from build123d import *

# Parameters (mm, degrees)
BOSS_EXTRUDE1_DEPTH     = 2.5
SKETCH2_W               = 2.5
SKETCH2_H               = 47.5
BOSS_EXTRUDE2_DEPTH     = 20
SKETCH3_W               = 2.5
SKETCH3_H               = 47.5
BOSS_EXTRUDE3_DEPTH     = 20
SKETCH4_W               = 17
SKETCH4_H               = 2.5
BOSS_EXTRUDE4_DEPTH     = 20.4
SKETCH5_W               = 1.5
SKETCH5_H               = 11
CUT_EXTRUDE1_DEPTH      = 48.5
SKETCH6_W               = 17
SKETCH6_H               = 2.5
BOSS_EXTRUDE5_DEPTH     = 20.4
SKETCH7_W               = 1.5
SKETCH7_H               = 11
CUT_EXTRUDE2_DEPTH      = 48.5
SKETCH8_W               = 2.7
SKETCH8_H               = 4.5
SKETCH9_W               = 2.7
SKETCH9_H               = 4.5
SKETCH10_W              = 2
SKETCH10_H              = 1.5
SKETCH11_W              = 2
SKETCH11_H              = 1.5
FILLET1_R               = 2
FILLET2_R               = 10
SKETCH13_R              = 3.6
SKETCH13_R_2            = 2.5
SKETCH13_R_3            = 1.5
CUT_EXTRUDE3_DEPTH      = 5.5
CUT_EXTRUDE3_DEPTH_BACK = 23.9


with BuildPart() as part:
    # Sketch1 → Boss-Extrude1 (new body)
    with BuildSketch(Plane(origin=(0, 0, 0), x_dir=(-1, 0, 0), z_dir=(0, 0, -1))):
        with BuildLine():
            Line((12, -20), (12, 32))
            Line((12, 32), (-12, 32))
            Line((-12, 32), (-12, -20))
            ThreePointArc((-12, -20), (0, -32), (12, -20))
        make_face()
    extrude(amount=-BOSS_EXTRUDE1_DEPTH)

    # Sketch2 → Boss-Extrude2 (add)
    with BuildSketch(Plane.ZY.offset(12)):
        with Locations((1.25, 8.25)):
            Rectangle(SKETCH2_W, SKETCH2_H)
    extrude(amount=BOSS_EXTRUDE2_DEPTH)

    # Sketch3 → Boss-Extrude3 (add)
    with BuildSketch(Plane(origin=(12, 0, 0), x_dir=(0, 0, -1), z_dir=(1, 0, 0))):
        with Locations((-1.25, 8.25)):
            Rectangle(SKETCH3_W, SKETCH3_H)
    extrude(amount=BOSS_EXTRUDE3_DEPTH)

    # Sketch4 → Boss-Extrude4 (add)
    with BuildSketch(Plane(origin=(0, 0, 0), x_dir=(-1, 0, 0), z_dir=(0, 0, -1))):
        with Locations((-23.5, -14.25)):
            Rectangle(SKETCH4_W, SKETCH4_H)
    extrude(amount=BOSS_EXTRUDE4_DEPTH)

    # Sketch5 → Cut-Extrude1 (cut, through all)
    with BuildSketch(Plane.XZ.offset(15.5)):
        with Locations((20.75, -14.9)):
            Rectangle(SKETCH5_W, SKETCH5_H)
    extrude(amount=-CUT_EXTRUDE1_DEPTH, mode=Mode.SUBTRACT)

    # Sketch6 → Boss-Extrude5 (add)
    with BuildSketch(Plane(origin=(0, 0, 0), x_dir=(-1, 0, 0), z_dir=(0, 0, -1))):
        with Locations((23.5, -14.25)):
            Rectangle(SKETCH6_W, SKETCH6_H)
    extrude(amount=BOSS_EXTRUDE5_DEPTH)

    # Sketch7 → Cut-Extrude2 (cut, through all)
    with BuildSketch(Plane.XZ.offset(15.5)):
        with Locations((-20.75, -14.9)):
            Rectangle(SKETCH7_W, SKETCH7_H)
    extrude(amount=-CUT_EXTRUDE2_DEPTH, mode=Mode.SUBTRACT)

    # Sketch8 → Revolve1 (revolve)
    with BuildSketch(Plane(origin=(0, 7.55, 0), x_dir=(1, 0, 0), z_dir=(0, 1, 0))):
        with Locations((10.85, -4.75)):
            Rectangle(SKETCH8_W, SKETCH8_H)
    revolve(axis=Axis((9.5, 7.55, 2.5), (0, 0, 1)))

    # Sketch9 → Revolve2 (revolve)
    with BuildSketch(Plane(origin=(0, 7.55, 0), x_dir=(1, 0, 0), z_dir=(0, 1, 0))):
        with Locations((24.85, -4.75)):
            Rectangle(SKETCH9_W, SKETCH9_H)
    revolve(axis=Axis((23.5, 7.55, 2.5), (0, 0, 1)))

    # Sketch10 → Revolve3 (revolve)
    with BuildSketch(Plane.XZ.offset(1.25)):
        with Locations((-18, -0.75)):
            Rectangle(SKETCH10_W, SKETCH10_H)
    revolve(axis=Axis((-19, -1.25, 0), (0, 0, -1)))

    # Sketch11 → Revolve4 (revolve)
    with BuildSketch(Plane.XZ.offset(-17.65)):
        with Locations((-0.5, -0.75)):
            Rectangle(SKETCH11_W, SKETCH11_H)
    revolve(axis=Axis((-1.5, 17.65, 0), (0, 0, -1)))

    # Fillet1
    fillet1_edges = [part.edges().sort_by_distance(p)[0] for p in [
        (32, -14.25, -20.4),
        (15, -14.25, -20.4),
        (-15, -14.25, -20.4),
        (-32, -14.25, -20.4),
    ]]
    fillet(fillet1_edges, radius=FILLET1_R)

    # Fillet2
    fillet2_edges = [part.edges().sort_by_distance(p)[0] for p in [
        (-32, 32, 1.25),
        (32, 32, 1.25),
    ]]
    fillet(fillet2_edges, radius=FILLET2_R)

    # Sketch13 → Cut-Extrude3 (cut, two sides)
    with BuildSketch(Plane.XY.offset(2.5)) as cut_extrude3_sk:
        with Locations((0, -20.1)):
            Circle(SKETCH13_R)
        with Locations((-20, 20.1)):
            Circle(SKETCH13_R_2)
        with Locations((-1.5, 17.65)):
            Circle(SKETCH13_R_3)
        with Locations((-19, -1.25)):
            Circle(SKETCH13_R_3)
        with Locations((9.5, 7.55)):
            Circle(SKETCH13_R_3)
        with Locations((23.5, 7.55)):
            Circle(SKETCH13_R_3)
    extrude(amount=CUT_EXTRUDE3_DEPTH, mode=Mode.SUBTRACT)
    extrude(cut_extrude3_sk.sketch, amount=-CUT_EXTRUDE3_DEPTH_BACK, mode=Mode.SUBTRACT)


solid = part.part
Design review of the part built by this model. Coordinates are the model's own, in mm. A direction names the side the tool comes from. Round coordinates to 2 decimals unless told otherwise and drop trailing zeros. Write each loop counter-clockwise with the first axis right and the second up, starting at its lowest first coordinate (ties: lowest second). Pieces come first, ordered by that corner, then holes. Notation, with made-up numbers: (9, 15.5) - (16, 15.5) arc R7 cw to (16, 23.5) - close; hole circle Ø11 at (21, 61). An arc over 180 degrees is marked (long way). Use a Markdown table: item, result. Add a question column.
1. Wall thickness on probe 1 along Y at (x, z) = (-20, 1.15); probe 2 along Y at (x, z) = (23.5, 5); probe 3 along X at (y, z) = (-14.5, -10): over which ranges is each line inside the solid? List them lowest first.
2. For faces 4 (the face through (21, -14, -9.4)), 5 (the face through (22, 6, 7)), 6 (the face through (-12, -18, 1)), 7 (the face through (12, -18, 1)), list the 3-axis set-ups (+Z, -Z, +X, -X, +Y, -Y) from which the entire face can be reached by the end or side of a thin tool; tool diameter is ignored.
3. We need section D-D (x = 23.5). State the section outline as (y, z) points.
4. We need section A-A (z = -14). State the section outline as (x, y) points, then the cut area to 3 significant figures.
5. We need section C-C (z = -4.5). State the section outline as (x, y) points.
6. Clearance check with flat-ended pins moving along their axes: pin 1 (2 mm diameter, centred on y = -18.5, z = 1, fed in from +X); pin 2 (19 mm diameter, centred on x = 4.5, y = -13.5, fed in from -Z); pin 3 (16 mm diameter, centred on x = -21.5, z = -11, fed in from -Y). State where each tip first meets the part, or that it passes through.
7. Mouldability with a two-part tool opening along Y and no side actions: class faces 1 (the face through (-0.47, -16.53, 1.27)), 2 (the face through (0, 32, 1)), 3 (the face through (26, -14, -20.4)) as +Y half, -Y half, draft (parallel to the pull), parting line (faces both ways), or undercut.
8. We need section B-B (y = -1.25). State the section outline as (x, z) points.
Output:
| question | item | result |
|---|---|---|
| 1 | probe 1 | y = -15.5 to -2.37, -0.13 to 17.6, 22.6 to 32 |
| 1 | probe 2 | y = 4.85 to 6.05, 9.05 to 10.25 |
| 1 | probe 3 | x = -32 to -21.5, -20 to -15, 15 to 20, 21.5 to 32 |
| 2 | face 4 | -Z, +Y, -Y |
| 2 | face 5 | +Z, +X, -X, +Y, -Y |
| 2 | face 6 | +Z, -Z, -X, -Y |
| 2 | face 7 | +Z, -Z, +X, -Y |
| 3 | outline | (-15.5, -20.4) - (-13, -20.4) - (-13, 0) - (6.05, 0) - (6.05, 7) - (4.85, 7) - (4.85, 2.5) - (-15.5, 2.5) - close; (9.05, 0) - (31.89, 0) - (31.89, 2.5) - (10.25, 2.5) - (10.25, 7) - (9.05, 7) - close |
| 4 | outline | (-32, -15.5) - (-21.5, -15.5) - (-21.5, -13) - (-32, -13) - close; (-20, -15.5) - (-15, -15.5) - (-15, -13) - (-20, -13) - close; (15, -15.5) - (20, -15.5) - (20, -13) - (15, -13) - close; (21.5, -15.5) - (32, -15.5) - (32, -13) - (21.5, -13) - close |
| 4 | area | 77.5 mm2 |
| 5 | outline | (-32, -15.5) - (-15, -15.5) - (-15, -13) - (-32, -13) - close; (15, -15.5) - (32, -15.5) - (32, -13) - (15, -13) - close |
| 6 | pin 1 | stops at x = 12 |
| 6 | pin 2 | stops at z = 0 |
| 6 | pin 3 | stops at y = -15.5 |
| 7 | face 1 | undercut |
| 7 | face 2 | +Y half |
| 7 | face 3 | draft |
| 8 | outline | (-32, 0) - (-21, 0) - (-21, -1.5) - (-20.5, -1.5) - (-20.5, 2.5) - (-32, 2.5) - close; (-17.5, -1.5) - (-17, -1.5) - (-17, 0) - (32, 0) - (32, 2.5) - (-17.5, 2.5) - close |
